Check sheet for the drawn part. Datum: minimum x, y, z corner. Units: mm. Round coordinates to 2 decimals unless told otherwise and drop trailing zeros. Loops run counter-clockwise (first coordinate to the right, second up) from the corner with the lowest first, then second, coordinate; pieces in that order, holes last.
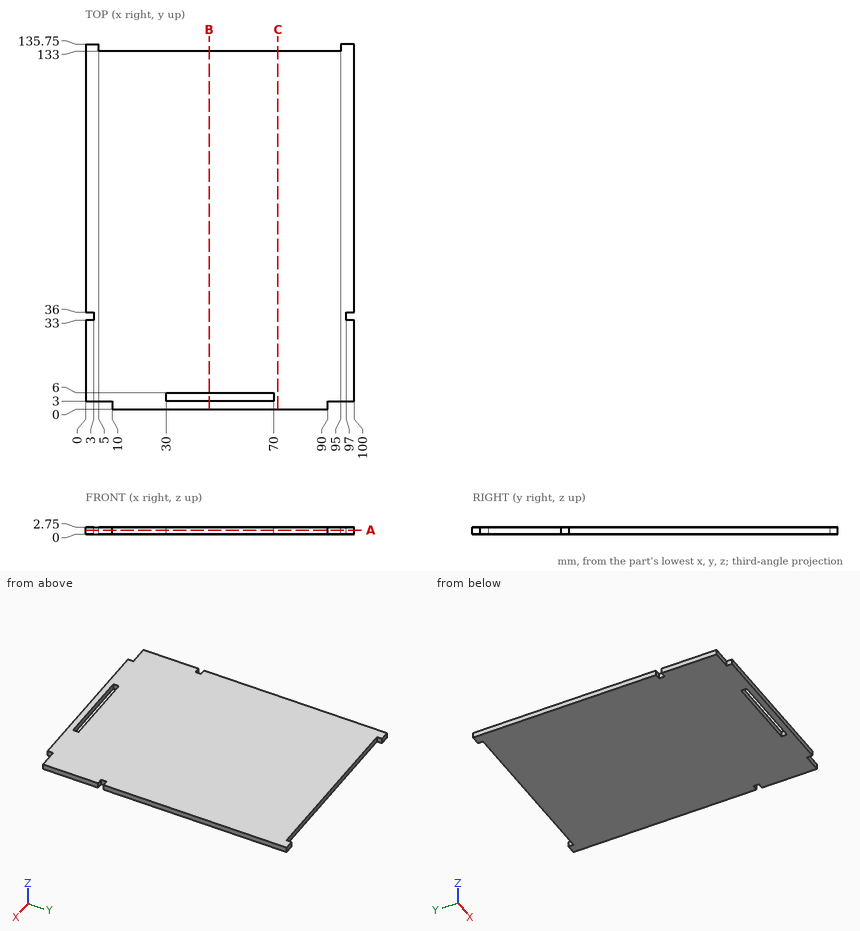
1. Section check A-A (z = 1.6). Enter the section's corners in (x, y).
2. Section check C-C (x = 71.5). Enter the section's corners in (y, z), then the cut area to 3 significant figures.
3. Section check B-B (x = 46). Enter the section's corners in (y, z), then the cut area to 4 significant figures.
4. Gauge pin test, flat ends, axial feed: P1, Ø1.4, axis at y = 35, z = 2, coming from the -X side; P2, Ø3, axis at x = 73.5, y = 93, coming from the -Z side; P3, Ø1.4, axis at x = 2.5, z = 1, coming from the -Y side; P4, Ø1.4, axis at y = 1, z = 1, coming from the +X side. Record the tip position at first contact, or that the pin passes through.
5. Scan lines: L1, parallel to Y at x = 65, z = 2; L2, parallel to Y at x = 81, z = 1.8; L3, parallel to Y at x = 94.5, z = 2.5. Record each from-to range of solid material in increasing order.
Taken from the geometry:
1. outline: (0, 3) - (10, 3) - (10, 0) - (90, 0) - (90, 3) - (100, 3) - (100, 33) - (97, 33) - (97, 36) - (100, 36) - (100, 135.75) - (95, 135.75) - (95, 133) - (5, 133) - (5, 135.75) - (0, 135.75) - (0, 36) - (3, 36) - (3, 33) - (0, 33) - close; hole (30, 3) - (70, 3) - (70, 6) - (30, 6) - close
2. outline: (0, 0) - (133, 0) - (133, 2.75) - (0, 2.75) - close
2. area: 366 mm2
3. outline: (0, 0) - (3, 0) - (3, 2.75) - (0, 2.75) - close; (6, 0) - (133, 0) - (133, 2.75) - (6, 2.75) - close
3. area: 357.5 mm2
4. P1: stops at x = 3
4. P2: stops at z = 0
4. P3: stops at y = 3
4. P4: stops at x = 90
5. L1: y = 0 to 3, 6 to 133
5. L2: y = 0 to 133
5. L3: y = 3 to 133
